from build123d import *

# Parameters (mm, degrees)
SKETCH1_W           = 30
SKETCH1_H           = 150
BOSS_EXTRUDE2_DEPTH = 10
SKETCH3_R           = 12.7
SKETCH3_R_2         = 9
CUT_EXTRUDE1_DEPTH  = 5
BOSS_EXTRUDE3_START = 20
SKETCH4_R           = 9
BOSS_EXTRUDE3_DEPTH = 20


with BuildPart() as part:
    # Sketch1 → Boss-Extrude2 (new body)
    with BuildSketch(Plane(origin=(0, 0, 0), x_dir=(1, 0, 0), z_dir=(0, 1, 0))):
        with Locations((-4.813074205, -44.932862191)):
            Rectangle(SKETCH1_W, SKETCH1_H)
    extrude(amount=BOSS_EXTRUDE2_DEPTH)

    # Sketch3 → Cut-Extrude1 (cut)
    with BuildSketch(Plane(origin=(0, 10, 0), x_dir=(1, 0, 0), z_dir=(0, 1, 0))):
        with Locations(Location((-4.813074205, -44.932862191, 0), (0, 0, 270))):
            Circle(SKETCH3_R)
        with Locations(Location((-4.813074205, -44.932862191, 0), (0, 0, 270))):
            Circle(SKETCH3_R_2, mode=Mode.SUBTRACT)
    extrude(amount=-CUT_EXTRUDE1_DEPTH, mode=Mode.SUBTRACT)

    # Sketch4 → Boss-Extrude3 (add)
    with BuildSketch(Plane(origin=(0, 10, 0), x_dir=(1, 0, 0), z_dir=(0, 1, 0)).offset(BOSS_EXTRUDE3_START)):
        with Locations(Location((-4.813074205, -44.932862191, 0), (0, 0, 270))):
            Circle(SKETCH4_R)
    extrude(amount=-BOSS_EXTRUDE3_DEPTH)


solid = part.part
Can you work these out from the model? Positions are in its coordinate system, mm. A direction names the side the tool comes from. Coordinates: 2 decimals unless noted, no trailing zeros. Write each loop counter-clockwise with the first axis right and the second up, starting at its lowest first coordinate (ties: lowest second). Pieces come first, ordered by that corner, then holes.
Q1. If we mould it in two halves opening along Z, with no side actions, what happens to faces 1 (the face through (-5, 5, 119.933)), 2 (the face through (-0.998, 7.535, 57.046)), 3 (the face through (-5, 0, 44))? For each: +Z half, -Z half, draft (parallel to the pull), parting line (faces both ways), or undercut.
Results found:
face 1: +Z half
face 2: undercut
face 3: draft
Q2. For P1, Ø10, axis at x = -15, y = 22.5, coming from the +Z side; P2, Ø1, axis at x = -11.5, y = 26, coming from the -Z side; P3, Ø8, axis at x = 5.5, z = 88.5, coming from the +Y side, each with a flat end and sliding along its axis, tell me the tip position at first contact or that it passes through.
Results found:
P1: stops at z = 52.29
P2: stops at z = 38.4
P3: stops at y = 10
Q3. Imagine slicing it at C-C, the plane y = 15. List the corners of the cut face in (x, z) for me, plus the area to 3 significant figures.
Results found:
outline: circle Ø18 at (-4.81, 44.93)
area: 254 mm2
Q4. Imagine slicing it at B-B, the plane z = 30.5. List the corners of the cut face in (x, y) for me.
Results found:
outline: (-19.81, 0) - (10.19, 0) - (10.19, 10) - (-19.81, 10) - close
Q5. Please list where these lines run through material, in increasing order: L1, parallel to Y at x = -8, z = 96.5; L2, parallel to Z at x = -4.75, y = 16.25; L3, parallel to Z at x = -13, y = 11.
Results found:
L1: y = 0 to 10
L2: z = 35.93 to 53.93
L3: z = 41.19 to 48.67
Q6. Imagine slicing it at D-D, the plane x = -9.5. List the corners of the cut face in (y, z) for me.
Results found:
outline: (0, -30.07) - (10, -30.07) - (10, 33.13) - (5, 33.13) - (5, 37.25) - (30, 37.25) - (30, 52.62) - (5, 52.62) - (5, 56.74) - (10, 56.74) - (10, 119.93) - (0, 119.93) - close
Q7. Which directions (+Z, -Z, +X, -X, +Y, -Y) give clear straight access to the entire face, cutting with the end or side of a thin tool? Please do faces 4 (the face through (-5, 30, 45)), 5 (the face through (4, 5, 48)).
Results found:
face 4: +Z, -Z, +X, -X, +Y
face 5: +Y
Q8. Imagine slicing it at A-A, the plane x = -1.25. List the corners of the cut face in (y, z) for me, plus the area to 3 significant figures.
Results found:
outline: (0, -30.07) - (10, -30.07) - (10, 32.74) - (5, 32.74) - (5, 36.67) - (30, 36.67) - (30, 53.2) - (5, 53.2) - (5, 57.12) - (10, 57.12) - (10, 119.93) - (0, 119.93) - close
area: 1,790 mm2
